Here's how the part is built. I have some questions about the finished solid (model axes, mm). A direction names the side the tool comes from. Coordinates: 2 decimals unless noted, no trailing zeros. Write each loop counter-clockwise with the first axis right and the second up, starting at its lowest first coordinate (ties: lowest second). Pieces come first, ordered by that corner, then holes.
```python
from build123d import *

# Parameters (mm, degrees)
ESQUISSE1_W             = 237.01
ESQUISSE1_H             = 19.49
BOSS_EXTRU_1_DEPTH      = 3
BOSS_EXTRU_2_DEPTH      = 3
ESQUISSE3_R             = 5
BOSS_EXTRU_3_DEPTH      = 10
ESQUISSE4_R             = 5
BOSS_EXTRU_4_DEPTH      = 10
ESQUISSE5_R             = 1.5
ENL_V_MAT_EXTRU_1_DEPTH = 10


with BuildPart() as part:
    # Esquisse1 → Boss.-Extru.1 (new body)
    with BuildSketch(Plane.XY):
        with Locations((59.527989935, 3.140717464)):
            Rectangle(ESQUISSE1_W, ESQUISSE1_H)
    extrude(amount=BOSS_EXTRU_1_DEPTH)

    # Esquisse2 → Boss.-Extru.2 (add)
    with BuildSketch(Plane(origin=(0, 10.885717464, 0), x_dir=(-1, 0, 0), z_dir=(0, 1, 0))):
        with BuildLine():
            Line((52.842010065, 3), (52.842010065, 18.31))
            ThreePointArc((52.842010065, 18.31), (41.727010065, 29.425), (30.612010065, 18.31))
            Line((30.612010065, 18.31), (30.612010065, 3))
            Line((30.612010065, 3), (52.842010065, 3))
        make_face()
        with BuildLine():
            Line((-171.897989935, 3), (-149.667989935, 3))
            Line((-149.667989935, 3), (-149.667989935, 18.31))
            ThreePointArc((-149.667989935, 18.31), (-160.782989935, 29.425), (-171.897989935, 18.31))
            Line((-171.897989935, 18.31), (-171.897989935, 3))
        make_face()
    extrude(amount=-BOSS_EXTRU_2_DEPTH)

    # Esquisse3 → Boss.-Extru.3 (add)
    with BuildSketch(Plane(origin=(0, 10.885717464, 0), x_dir=(-1, 0, 0), z_dir=(0, 1, 0))):
        with Locations((41.727010065, 18.31)):
            Circle(ESQUISSE3_R)
    extrude(amount=BOSS_EXTRU_3_DEPTH)

    # Esquisse4 → Boss.-Extru.4 (add)
    with BuildSketch(Plane(origin=(0, 10.885717464, 0), x_dir=(-1, 0, 0), z_dir=(0, 1, 0))):
        with Locations((-160.782989935, 18.31)):
            Circle(ESQUISSE4_R)
    extrude(amount=BOSS_EXTRU_4_DEPTH)

    # Esquisse5 → Enlèv. mat.-Extru.1 (cut)
    with BuildSketch(Plane.XY.offset(3)):
        with Locations((-23.977010065, 7.885717464)):
            Circle(ESQUISSE5_R)
        with Locations((143.032989935, 7.885717464)):
            Circle(ESQUISSE5_R)
    extrude(amount=-ENL_V_MAT_EXTRU_1_DEPTH, mode=Mode.SUBTRACT)


solid = part.part
```
1) I need wall thicknesses on probe 1 along X at (y, z) = (10.25, 18.5); probe 2 along Z at (x, y) = (164.5, -3); probe 3 along X at (y, z) = (10.75, 20.75). Which ranges of each line are inside material? Lowest first, please.
Values follow:
probe 1: x = -52.84 to -30.61, 149.67 to 171.9
probe 2: z = 0 to 3
probe 3: x = -52.57 to -30.88, 149.94 to 171.63
2) Imagine slicing it at D-D on z = 27. Please give me the cut outline in (x, y), then the cut area to 3 significant figures.
Values follow:
outline: (-48.66, 7.89) - (-34.8, 7.89) - (-34.8, 10.89) - (-48.66, 10.89) - close; (153.85, 7.89) - (167.71, 7.89) - (167.71, 10.89) - (153.85, 10.89) - close
area: 83.2 mm2
3) Imagine slicing it at A-A on z = 8.75. Please give me the cut outline in (x, y).
Values follow:
outline: (-52.84, 7.89) - (-30.61, 7.89) - (-30.61, 10.89) - (-52.84, 10.89) - close; (149.67, 7.89) - (171.9, 7.89) - (171.9, 10.89) - (149.67, 10.89) - close
4) Imagine slicing it at C-C on x = 163. Please give me the cut outline in (y, z).
Values follow:
outline: (-6.6, 0) - (12.89, 0) - (12.89, 3) - (10.89, 3) - (10.89, 13.83) - (20.89, 13.83) - (20.89, 22.79) - (10.89, 22.79) - (10.89, 29.2) - (7.89, 29.2) - (7.89, 3) - (-6.6, 3) - close
5) Will these pins go through, and if not, where does the flat tip stop? pin 1 (10 mm diameter, centred on x = 141.5, y = -0.5, fed in from +Z); pin 2 (3.5 mm diameter, centred on y = 8.5, z = 13.5, fed in from -X); pin 3 (0.9 mm diameter, centred on y = 9, z = 11, fed in from +X); pin 4 (5 mm diameter, centred on x = 126.5, y = -2, fed in from -Z).
Values follow:
pin 1: stops at z = 3
pin 2: stops at x = -52.84
pin 3: stops at x = 171.9
pin 4: stops at z = 0
6) On a 3-axis mill with a long thin cutter (end or side, diameter ignored), from which of +Z, -Z, +X, -X, +Y, -Y can I reach the whole of each face in a straight line? I mean faces 1 (the face through (-41.971, 9.407, 29.422)), 2 (the face through (165.78, 15.82, 18.53)), 3 (the face through (-42, 7.886, 16)). Say none if no direction works.
Values follow:
face 1: +Z, +Y, -Y
face 2: +Y
face 3: +Z, +X, -X, -Y
7) Imagine slicing it at B-B on y = 16.25. Please give me the cut outline in (x, z).
Values follow:
outline: circle Ø10 at (-41.73, 18.31); circle Ø10 at (160.78, 18.31)
